For this review, take the finished solid that the model builds, in its own axes (mm). A direction names the side the tool comes from. Give positions to 0.01 mm unless a question says otherwise; leave off trailing zeros. Order: outer loops, then holes, each group sorted by start corner. A loop starts at its lowest first (then second) coordinate and runs counter-clockwise, first axis right, second up. Notation, with made-up numbers: M -32,89.5 L 11,89.5 A8 ccw 11,96.5 Z; hole C 87.5,45.5 d3. An arc over 180 degrees is marked long. Answer as CSV lines item,"result". Start each with the question number.
1. We need section C-C, the plane z = -15.5. Give the boundary of the cut face in (x, y).
2. For line 1 along X through (y, z) = (2, 15); line 2 along X through (y, z) = (2.2, 0); line 3 along Z through (x, y) = (3.5, 23), list the stretches that pass through material, from the lowest coordinate up.
3. Machinability: for faces 5 (the flat face through (0, 14, 42)), 6 (the cylindrical face through (35.72, 4.93, -41.19)), 7 (the cylindrical face through (-35.72, 4.93, 41.19)), 8 (the cylindrical face through (41.19, 4.93, 35.72)), 9 (the cylindrical face through (-0.1, 38.5, -45)), which of the approach directions +Z, -Z, +X, -X, +Y, -Y give a long, thin tool a straight path to every point of the face, cutting with its end or side? Answer none if there is none.
4. We need section B-B, the plane x = 0. State how many separate pieces and enclosed holes the cut face has, and give its area (3 significant figures).
5. Mouldability with a two-part tool opening along X and no side actions: class faces 1 (the cylindrical face through (-41.19, 4.93, -35.72)), 2 (the cylindrical face through (0.33, 1.521, 22.507)), 3 (the flat face through (-8, 38, 39.5)), 4 (the cylindrical face through (0.9, 1.52, 2.86)) as pulls with the +X half, pulls with the -X half, needs draft (parallel to the pull), parting line crosses it, or undercut.
6. Clearance check with flat-ended pins moving along their axes: P1, Ø5, axis at y = 25.5, z = 5, coming from the +X side; P2, Ø10, axis at x = -7.5, y = 30, coming from the +Z side; P3, Ø12, axis at x = -25.98, z = 15, coming from the +Y side; P4, Ø12, axis at x = 16, z = -16.5, coming from the +Y side. State where each tip first meets the part, or that it passes through.
7. We need section D-D, the plane y = 16. Give the boundary of the cut face in (x, z), and give its area (3 significant figures).
8. We need section A-A, the plane y = 41.5. Give the boundary of the cut face in (x, z).
from build123d import *

# Parameters (mm, degrees)
BOSS_EXTRUDE1_DEPTH            = 40
SHELL1_T                       = -3
SKETCH2_R                      = 3
SKETCH2_R_2                    = 7.5
CUT_EXTRUDE1_DEPTH             = 3
SKETCH3_R                      = 3
BOSS_EXTRUDE2_DEPTH            = 10
FILLET1_R                      = 5
CIRPATTERN1_OUTLINE_R          = 3
CIRPATTERN1_DEPTH              = 10
SKETCH4_R                      = 1.75
BOSS_EXTRUDE3_DEPTH            = 17.5
FILLET2_R                      = 5
FILLET3_R                      = 5
SKETCH5_R                      = 3
CUT_EXTRUDE2_DEPTH             = 4
CUT_EXTRUDE3_DEPTH             = 4
CUT_EXTRUDE3_DEPTH_BACK        = 4
SKETCH6_R                      = 3
SKETCH7_W                      = 10
SKETCH7_H                      = 20
CUT_EXTRUDE4_DEPTH             = 7.5
SKETCH9_W                      = 10
SKETCH9_H                      = 25
CUT_EXTRUDE6_DEPTH             = 7.5
SKETCH8_W                      = 11
SKETCH8_H                      = 12
CUT_EXTRUDE7_DEPTH             = 24
CUT_EXTRUDE7_DIRECTION_2_REACH = 92.847


# Read off the part's stored shape, not the designer's step: CirPattern1
with BuildPart() as part:
    # Sketch1 → Boss-Extrude1 (new body)
    with BuildSketch(Plane(origin=(0, 0, 0), x_dir=(1, 0, 0), z_dir=(0, 1, 0))):
        with BuildLine():
            Line((-17.5, 42), (17.5, 42))
            ThreePointArc((17.5, 42), (45.5, 0), (17.5, -42))
            Line((17.5, -42), (-17.5, -42))
            ThreePointArc((-17.5, -42), (-45.5, 0), (-17.5, 42))
        make_face()
    extrude(amount=BOSS_EXTRUDE1_DEPTH)

    # Shell1
    shell1_openings = [part.faces().sort_by_distance(p)[0] for p in [
        (0, 40, 0),
    ]]
    offset(amount=SHELL1_T, openings=shell1_openings, kind=Kind.INTERSECTION)

    # Sketch2 → Cut-Extrude1 (cut)
    with BuildSketch(Plane(origin=(0, 3, 0), x_dir=(1, 0, 0), z_dir=(0, 1, 0))):
        with Locations(Location((0, 0, 0), (0, 0, 270))):
            Circle(SKETCH2_R)
        with Locations(Location((0, 30, 0), (0, 0, 270))):
            Circle(SKETCH2_R_2)
        with Locations(Location((25.980762114, 15, 0), (0, 0, 270))):
            Circle(SKETCH2_R_2)
        with Locations(Location((25.980762114, -15, 0), (0, 0, 270))):
            Circle(SKETCH2_R_2)
        with Locations(Location((0, -30, 0), (0, 0, 270))):
            Circle(SKETCH2_R_2)
        with Locations(Location((-25.980762114, -15, 0), (0, 0, 270))):
            Circle(SKETCH2_R_2)
        with Locations(Location((-25.980762114, 15, 0), (0, 0, 270))):
            Circle(SKETCH2_R_2)
    extrude(amount=-CUT_EXTRUDE1_DEPTH, mode=Mode.SUBTRACT)

    # Sketch3 → Boss-Extrude2 (add)
    with BuildSketch(Plane.XZ):
        with BuildLine():
            Line((-35.850313806, 28.017940681), (-41.507168056, 35.850313806))
            Line((-41.507168056, 35.850313806), (-41.507168056, 41.507168056))
            Line((-41.507168056, 41.507168056), (-35.850313806, 41.507168056))
            Line((-35.850313806, 41.507168056), (-28.017940681, 35.850313806))
            ThreePointArc((-28.017940681, 35.850313806), (-32.173358544, 32.173358544), (-35.850313806, 28.017940681))
        make_face()
        with Locations(Location((-35.850313806, 35.850313806, 0), (0, 0, 270))):
            Circle(SKETCH3_R, mode=Mode.SUBTRACT)
    extrude(amount=-BOSS_EXTRUDE2_DEPTH)

    # Fillet1
    # the kernel refuses this fillet: 5 mm, written as the material it adds along each edge
    with BuildSketch(Plane(origin=(-28.017940681, 0, 35.850313806), x_dir=(0.8105373937900577, 0, 0.585686890128182), z_dir=(0, 1, 0))) as fillet1_piece_1:
        with BuildLine():
            CenterArc((3.613249721, -4.996457194), FILLET1_R, 92.157009058, 69.532849002)
            Line((-1.133599694, -3.425654648), (0, 0))
            ThreePointArc((0, 0), (1.712529816, -0.032239536), (3.425059631, 0))
        make_face()
    extrude(amount=10)
    with BuildSketch(Plane(origin=(-35.850313806, 0, 28.017940681), x_dir=(-0.5856868901281832, 0, -0.8105373937900566), z_dir=(0, 1, 0))) as fillet1_piece_2:
        with BuildLine():
            CenterArc((3.613249721, 4.996457194), FILLET1_R, 198.31014194, 69.532849002)
            Line((-1.133599694, 3.425654648), (0, 0))
            ThreePointArc((0, 0), (1.712529816, 0.032239536), (3.425059631, 0))
        make_face()
    extrude(amount=10)
    # the kernel refuses this fillet: 5 mm, written as the material it takes off along each edge
    with BuildSketch(Plane(origin=(-41.507168056, -12.5, 41.507168056), x_dir=(1, 0, 0), z_dir=(0, 1, 0))) as fillet1_2_piece_1:
        with BuildLine():
            CenterArc((FILLET1_R, FILLET1_R), FILLET1_R, 180, 90)
            Line((0, FILLET1_R), (0, 0))
            Line((0, 0), (FILLET1_R, 0))
        make_face()
    extrude(amount=35, mode=Mode.SUBTRACT)
    with BuildSketch(Plane(origin=(-35.850313806, -4.042007545, 41.507168056), x_dir=(0.8106723345515203, 0, -0.5855000990544645), z_dir=(0, 1, 0)), Plane(origin=(-41.507168056, -4.042007545, 35.850313806), x_dir=(0, 0, 1), z_dir=(0, 1, 0))) as fillet1_2_piece_2:
        with BuildLine():
            CenterArc((FILLET1_R * 0.323360603618, FILLET1_R), FILLET1_R, 234.161672423, 35.838327577)
            Line((-FILLET1_R * 0.262139495437, FILLET1_R * 0.189327665448), (0, 0))
            Line((0, 0), (FILLET1_R * 0.323360603618, 0))
        make_face()
    extrude(amount=18.08401509, mode=Mode.SUBTRACT)

    # CirPattern1 outline → CirPattern1 (add)
    # profile 1 of 3: a face of its own
    with BuildSketch(Plane(origin=(0, 0, 0), x_dir=(1, 0, 0), z_dir=(0, 1, 0))):
        with BuildLine():
            ThreePointArc((35.850313806, -28.017940681), (32.173358544, -32.173358544), (28.017940681, -35.850313806))
            Line((28.017940681, -35.850313806), (34.539616329, -40.560529728))
            ThreePointArc((34.539616329, -40.560529728), (35.701909685, -41.185206507), (36.98714244, -41.484077196))
            ThreePointArc((36.98714244, -41.484077196), (40.042701962, -40.042701962), (41.484077196, -36.98714244))
            ThreePointArc((41.484077196, -36.98714244), (41.185206507, -35.701909685), (40.560529728, -34.539616329))
            Line((40.560529728, -34.539616329), (35.850313806, -28.017940681))
        make_face()
        with Locations((35.850313806, -35.850313806)):
            Circle(CIRPATTERN1_OUTLINE_R, mode=Mode.SUBTRACT)
    # profile 2 of 3: a face of its own
    with BuildSketch(Plane(origin=(0, 0, 0), x_dir=(1, 0, 0), z_dir=(0, 1, 0))):
        with BuildLine():
            ThreePointArc((28.017940681, 35.850313806), (32.173358544, 32.173358544), (35.850313806, 28.017940681))
            Line((35.850313806, 28.017940681), (40.560529728, 34.539616329))
            ThreePointArc((40.560529728, 34.539616329), (41.185206507, 35.701909685), (41.484077196, 36.98714244))
            ThreePointArc((41.484077196, 36.98714244), (40.042701962, 40.042701962), (36.98714244, 41.484077196))
            ThreePointArc((36.98714244, 41.484077196), (35.701909685, 41.185206507), (34.539616329, 40.560529728))
            Line((34.539616329, 40.560529728), (28.017940681, 35.850313806))
        make_face()
        with Locations((35.850313806, 35.850313806)):
            Circle(CIRPATTERN1_OUTLINE_R, mode=Mode.SUBTRACT)
    # profile 3 of 3: a face of its own
    with BuildSketch(Plane(origin=(0, 0, 0), x_dir=(1, 0, 0), z_dir=(0, 1, 0))):
        with BuildLine():
            ThreePointArc((-25.241801774, 37.85632633), (-28.109161878, 37.01723716), (-30.94312664, 37.963000518))
            Line((-30.94312664, 37.963000518), (-34.539616329, 40.560529728))
            ThreePointArc((-34.539616329, 40.560529728), (-35.701909685, 41.185206507), (-36.98714244, 41.484077196))
            ThreePointArc((-36.98714244, 41.484077196), (-40.042701962, 40.042701962), (-41.484077196, 36.98714244))
            ThreePointArc((-41.484077196, 36.98714244), (-41.185206507, 35.701909685), (-40.560529728, 34.539616329))
            Line((-40.560529728, 34.539616329), (-37.963000518, 30.94312664))
            ThreePointArc((-37.963000518, 30.94312664), (-37.01723716, 28.109161878), (-37.85632633, 25.241801774))
            ThreePointArc((-37.85632633, 25.241801774), (-32.173358544, 32.173358544), (-25.241801774, 37.85632633))
        make_face()
        with Locations((-35.850313806, 35.850313806)):
            Circle(CIRPATTERN1_OUTLINE_R, mode=Mode.SUBTRACT)
    extrude(amount=CIRPATTERN1_DEPTH)

    # Sketch4 → Boss-Extrude3 (add, symmetric)
    with BuildSketch(Plane(origin=(0, 0, 0), x_dir=(0, 0, -1), z_dir=(1, 0, 0))):
        with BuildLine():
            Line((-42, 30), (-47.598076211, 38.5))
            Line((-47.598076211, 38.5), (-47.598076211, 40))
            ThreePointArc((-47.598076211, 40), (-45, 44.5), (-42.401923789, 40))
            Line((-42.401923789, 40), (-42, 40))
            Line((-42, 40), (-42, 30))
        make_face()
        with Locations((-45, 41.5)):
            Circle(SKETCH4_R, mode=Mode.SUBTRACT)
    boss_extrude3 = extrude(amount=BOSS_EXTRUDE3_DEPTH, both=True)

    # Fillet2
    fillet2_edges = [part.edges().sort_by_distance(p)[0] for p in [
        (0, 30, 42),
        (0, 38.5, 47.598076211),
    ]]
    fillet(fillet2_edges, radius=FILLET2_R)

    # Mirror1: Boss-Extrude3 across plane
    add(boss_extrude3.mirror(Plane.XY))

    # Fillet3
    fillet3_edges = [part.edges().sort_by_distance(p)[0] for p in [
        (0, 30, -42),
        (0, 38.5, -47.598076211),
    ]]
    fillet(fillet3_edges, radius=FILLET3_R)

    # Sketch5 → Cut-Extrude2 (cut)
    with BuildSketch(Plane(origin=(17.5, 0, 0), x_dir=(0, 0, -1), z_dir=(1, 0, 0))):
        with Locations((-45, 41.5)):
            Circle(SKETCH5_R)
    extrude(amount=-CUT_EXTRUDE2_DEPTH, mode=Mode.SUBTRACT)

    # Sketch6 → Cut-Extrude3 (cut, two sides: drawn at the far end of the back side and taken through both)
    with BuildSketch(Plane(origin=(0, 0, 0), x_dir=(0, 0, -1), z_dir=(1, 0, 0)).offset(-CUT_EXTRUDE3_DEPTH_BACK)):
        with Locations((45, 41.5)):
            Circle(SKETCH6_R)
    extrude(amount=CUT_EXTRUDE3_DEPTH + CUT_EXTRUDE3_DEPTH_BACK, mode=Mode.SUBTRACT)

    # Sketch7 → Cut-Extrude4 (cut)
    with BuildSketch(Plane.ZY.offset(17.5)):
        with Locations((-47, 38.501412431)):
            Rectangle(SKETCH7_W, SKETCH7_H)
    extrude(amount=-CUT_EXTRUDE4_DEPTH, mode=Mode.SUBTRACT)

    # Sketch9 → Cut-Extrude6 (cut)
    with BuildSketch(Plane(origin=(17.5, 0, 0), x_dir=(0, 0, -1), z_dir=(1, 0, 0))):
        with Locations((47, 38.001412431)):
            Rectangle(SKETCH9_W, SKETCH9_H)
    extrude(amount=-CUT_EXTRUDE6_DEPTH, mode=Mode.SUBTRACT)

    # Sketch8 → Cut-Extrude7 (cut)
    with BuildSketch(Plane.ZY.offset(17.5)):
        with Locations((45, 41.5)):
            Rectangle(SKETCH8_W, SKETCH8_H)
    extrude(amount=-CUT_EXTRUDE7_DEPTH, mode=Mode.SUBTRACT)

    # Sketch8 → Cut-Extrude7 direction 2 (cut, up to next)
    with BuildSketch(Plane.ZY.offset(17.5), mode=Mode.PRIVATE) as cut_extrude7_direction_2_sk1:
        with Locations((45, 41.5)):
            Rectangle(SKETCH8_W, SKETCH8_H)
    cut_extrude7_direction_2_tool1 = extrude(cut_extrude7_direction_2_sk1.sketch, amount=CUT_EXTRUDE7_DIRECTION_2_REACH, mode=Mode.PRIVATE) & part.part
    add(cut_extrude7_direction_2_tool1.solids().sort_by_distance((-17.5, 41.5, 45))[0], mode=Mode.SUBTRACT)


solid = part.part
Result set:
1,outline,"M -42.78,0 L -33.46,0 L -33.46,3 L -39.57,3 L -39.57,40 L -42.78,40 Z; M -18.5,0 L 18.5,0 L 18.5,3 L -18.5,3 Z; M 33.46,0 L 42.78,0 L 42.78,40 L 39.57,40 L 39.57,3 L 33.46,3 Z"
2,line 1,"-42.96 to -33.48, -18.48 to 18.48, 33.48 to 42.96"
2,line 2,"-45.5 to -3, 3 to 45.5"
2,line 3,"-42 to -39, 39 to 42"
3,face 5,"+Z, +X, -X, -Y"
3,face 6,"-Z, +Y, -Y"
3,face 7,"+Z, +Y, -Y"
3,face 8,"+X, +Y, -Y"
3,face 9,"+Y"
4,separate pieces,"4"
4,enclosed holes,"0"
4,area,"392 mm2"
5,face 1,"pulls with the -X half"
5,face 2,"undercut"
5,face 3,"needs draft"
5,face 4,"undercut"
6,P1,"x = 45.43"
6,P2,"z = 45.29"
6,P3,"through"
6,P4,"y = 3"
7,outline,"M -17.5,-42 L 17.5,-42 A45.5 ccw 17.5,42 L -17.5,42 A45.5 ccw Z; hole M -16.89,-39 L 16.89,-39 A42.5 ccw 16.89,39 L -16.89,39 A42.5 ccw Z"
7,area,"824 mm2"
8,outline,"M -10,-48 L -4,-48 L -4,-46.75 L -10,-46.75 Z; M -10,-43.25 L -4,-43.25 L -4,-42 L -10,-42 Z; M 4,-48 L 10,-48 L 10,-46.75 L 4,-46.75 Z; M 4,-43.25 L 10,-43.25 L 10,-42 L 4,-42 Z; M 6.5,42 L 13.5,42 L 13.5,43.25 L 6.5,43.25 Z; M 6.5,46.75 L 13.5,46.75 L 13.5,48 L 6.5,48 Z"
